from build123d import *

# Parameters (mm, degrees)
SKETCH_1_R               = 113.5
SKETCH_1_R_2             = 17.5
EXTRUDE_1_DEPTH          = 1.5
CUT_EXTRUDE_1_DEPTH      = 2.5
CUT_EXTRUDE_2_DEPTH      = 2.5
PATTERN_CIRCULAR_1_COUNT = 3


with BuildPart() as part:
    # Эскиз1 → Бобышка-Вытянуть1 (new body)
    with BuildSketch(Plane(origin=(0, 0, 0), x_dir=(0, 0, -1), z_dir=(1, 0, 0))):
        Circle(SKETCH_1_R)
        Circle(SKETCH_1_R_2, mode=Mode.SUBTRACT)
    extrude(amount=EXTRUDE_1_DEPTH)

    # Эскиз2 → Вырез-Вытянуть1 (cut, through all)
    with BuildSketch(Plane.ZY):
        with BuildLine():
            Line((-16, 101.749692874), (-16, 46.353695472))
            Line((-16, 46.353695472), (-7.339745962, 41.353695472))
            ThreePointArc((-7.339745962, 41.353695472), (0, 42), (7.339745962, 41.353695472))
            Line((7.339745962, 41.353695472), (16, 46.353695472))
            Line((16, 46.353695472), (16, 101.749692874))
            ThreePointArc((16, 101.749692874), (0, 103), (-16, 101.749692874))
        make_face()
        with BuildLine():
            Line((96.117818856, -37.018439977), (48.143477838, -9.320441276))
            Line((48.143477838, -9.320441276), (39.4832238, -14.320441276))
            ThreePointArc((39.4832238, -14.320441276), (36.373066959, -21), (32.143477838, -27.033254197))
            Line((32.143477838, -27.033254197), (32.143477838, -37.033254197))
            Line((32.143477838, -37.033254197), (80.117818856, -64.731252898))
            ThreePointArc((80.117818856, -64.731252898), (89.20061659, -51.5), (96.117818856, -37.018439977))
        make_face()
        with BuildLine():
            Line((-80.117818856, -64.731252898), (-32.143477838, -37.033254197))
            Line((-32.143477838, -37.033254197), (-32.143477838, -27.033254197))
            ThreePointArc((-32.143477838, -27.033254197), (-36.373066959, -21), (-39.4832238, -14.320441276))
            Line((-39.4832238, -14.320441276), (-48.143477838, -9.320441276))
            Line((-48.143477838, -9.320441276), (-96.117818856, -37.018439977))
            ThreePointArc((-96.117818856, -37.018439977), (-89.20061659, -51.5), (-80.117818856, -64.731252898))
        make_face()
    extrude(amount=-CUT_EXTRUDE_1_DEPTH, mode=Mode.SUBTRACT)

    # Эскиз3 → Вырез-Вытянуть2 (cut, through all)
    with BuildSketch(Plane.ZY):
        with BuildLine():
            ThreePointArc((-78.144774985, -73.821705091), (-76.013978978, -76.013978978), (-73.821705091, -78.144774985))
            ThreePointArc((-73.821705091, -78.144774985), (-70.994421741, -78.064345778), (-71.074850948, -75.237062428))
            ThreePointArc((-71.074850948, -75.237062428), (-73.185551853, -73.185551853), (-75.237062428, -71.074850948))
            ThreePointArc((-75.237062428, -71.074850948), (-78.064345778, -70.994421741), (-78.144774985, -73.821705091))
        make_face()
        with BuildLine():
            ThreePointArc((-43.946014694, -98.107073101), (-41.138468979, -99.317049745), (-38.297651676, -100.446701669))
            ThreePointArc((-38.297651676, -100.446701669), (-35.716361381, -99.290440274), (-36.872622776, -96.709149979))
            ThreePointArc((-36.872622776, -96.709149979), (-39.60773525, -95.621531615), (-42.310814148, -94.456577358))
            ThreePointArc((-42.310814148, -94.456577358), (-44.953662293, -95.464224956), (-43.946014694, -98.107073101))
        make_face()
        with BuildLine():
            ThreePointArc((-3.056872038, -107.456528575), (0, -107.5), (3.056872038, -107.456528575))
            ThreePointArc((3.056872038, -107.456528575), (4.999191229, -105.400465308), (2.943127962, -103.458146116))
            ThreePointArc((2.943127962, -103.458146116), (0, -103.5), (-2.943127962, -103.458146116))
            ThreePointArc((-2.943127962, -103.458146116), (-4.999191229, -105.400465308), (-3.056872038, -107.456528575))
        make_face()
        with BuildLine():
            ThreePointArc((43.946014694, -98.107073101), (41.138468979, -99.317049745), (38.297651676, -100.446701669))
            ThreePointArc((38.297651676, -100.446701669), (35.716361381, -99.290440274), (36.872622776, -96.709149979))
            ThreePointArc((36.872622776, -96.709149979), (39.60773525, -95.621531615), (42.310814148, -94.456577358))
            ThreePointArc((42.310814148, -94.456577358), (44.953662293, -95.464224956), (43.946014694, -98.107073101))
        make_face()
        with BuildLine():
            ThreePointArc((78.144774985, -73.821705091), (76.013978978, -76.013978978), (73.821705091, -78.144774985))
            ThreePointArc((73.821705091, -78.144774985), (70.994421741, -78.064345778), (71.074850948, -75.237062428))
            ThreePointArc((71.074850948, -75.237062428), (73.185551853, -73.185551853), (75.237062428, -71.074850948))
            ThreePointArc((75.237062428, -71.074850948), (78.064345778, -70.994421741), (78.144774985, -73.821705091))
        make_face()
    cut_extrude_2 = extrude(amount=-CUT_EXTRUDE_2_DEPTH, mode=Mode.SUBTRACT)

    # Круговой массив1: Вырез-Вытянуть2 ×3 about axis
    pattern_circular_1_axis = Axis((0, 0, 0), (1, 0, 0))
    for i in range(1, PATTERN_CIRCULAR_1_COUNT):
        add(cut_extrude_2.rotate(pattern_circular_1_axis, i * 360 / PATTERN_CIRCULAR_1_COUNT), mode=Mode.SUBTRACT)


solid = part.part
Here's how the part is built. I have some questions about the finished solid (model axes, mm). A direction names the side the tool comes from. Coordinates: 2 decimals unless noted, no trailing zeros. Write each loop counter-clockwise with the first axis right and the second up, starting at its lowest first coordinate (ties: lowest second). Pieces come first, ordered by that corner, then holes.
Item 1: I want a section at D-D on x = 1.25. Count the separate pieces of the cut face and the enclosed holes in it, and give its area (3 significant figures).
Item 2: If I drill on line 1 (Y direction, x = 0.5, z = 0); line 2 (Z direction, x = 1.35, y = -37.5); line 3 (Y direction, x = 0.95, z = -9), over which ranges is the centre line in solid material (lowest first)?
Item 3: I want a section at C-C on y = -47.5. Write out the boundary of the cut face in (x, z).
Item 4: I want a section at B-B on y = 0. Write out the boundary of the cut face in (x, z), and give its area (3 significant figures).
Item 5: On a 3-axis mill with a long thin cutter (end or side, diameter ignored), from which of +Z, -Z, +X, -X, +Y, -Y can I reach the whole of each face in a straight line? I mean faces 1 (the flat face through (0, -24, 2)), 2 (the flat face through (0.74, -51.08, -56.47)). Say none if no direction works.
Item 6: If we mould it in two halves opening along Z, with no side actions, what happens to faces 3 (the cylindrical face through (0.74, 76.709, 83.654)), 4 (the flat face through (1.5, -24, 2)), 5 (the flat face through (0.74, -11.855, -43.753))? For each: +Z half, -Z half, draft (parallel to the pull), parting line (faces both ways), or undercut.
Item 7: I want a section at A-A on z = 0. Write out the boundary of the cut face in (x, y), and give its area (4 significant figures).
Item 8: Will these pins go through, and if not, where does the flat tip stop? pin 1 (10 mm diameter, centred on y = -19.5, z = 40.5, fed in from -X); pin 2 (0.8 mm diameter, centred on x = 0.5, y = 84, fed in from -Z).
Findings below:
1. separate pieces: 1
1. enclosed holes: 19
1. area: 33,200 mm2
2. line 1: y = -113.5 to -107.5, -103.5 to -17.5, 17.5 to 42, 103 to 113.5
2. line 2: z = -107.13 to -95.93, -32.95 to 32.95, 95.93 to 107.13
2. line 3: y = -113.14 to -15.01, 15.01 to 42.31, 102.61 to 113.14
3. outline: (0, -103.08) - (1.5, -103.08) - (1.5, -91.39) - (0, -91.39) - close; (0, -50.27) - (1.5, -50.27) - (1.5, 50.27) - (0, 50.27) - close; (0, 91.39) - (1.5, 91.39) - (1.5, 103.08) - (0, 103.08) - close
4. outline: (0, -113.5) - (1.5, -113.5) - (1.5, -17.5) - (0, -17.5) - close; (0, 17.5) - (1.5, 17.5) - (1.5, 113.5) - (0, 113.5) - close
4. area: 288 mm2
5. face 1: +Z, -Z, -X, +Y, -Y
5. face 2: +X, -X
6. face 3: parting line
6. face 4: draft
6. face 5: undercut
7. outline: (0, -113.5) - (1.5, -113.5) - (1.5, -107.5) - (0, -107.5) - close; (0, -103.5) - (1.5, -103.5) - (1.5, -17.5) - (0, -17.5) - close; (0, 17.5) - (1.5, 17.5) - (1.5, 42) - (0, 42) - close; (0, 103) - (1.5, 103) - (1.5, 113.5) - (0, 113.5) - close
7. area: 190.5 mm2
8. pin 1: stops at x = 0
8. pin 2: stops at z = -76.77
